Read the model definition and answer for the solid it produces. Units are mm, in the model's axes. A direction names the side the tool comes from. Give positions to 0.01 mm unless a question says otherwise; leave off trailing zeros. Order: outer loops, then holes, each group sorted by start corner. A loop starts at its lowest first (then second) coordinate and runs counter-clockwise, first axis right, second up. Notation, with made-up numbers: (88, -26) - (135, -26) arc R23 cw to (135, 5) - close; hole circle Ø2 at (11, 52.25). An arc over 180 degrees is marked (long way). Return JSON: item names as keys, results as strings.
```python
from build123d import *

# Parameters (mm, degrees)
F0_R     = 7.7179968939
F1_DEPTH = 38.1
F2_W     = 6.3499980524
F2_H     = 3.8099980524
F2_H_2   = 5.3974985393
F3_DEPTH = 12.7
F4_W     = 79.248
F4_H     = 25.4
F5_DEPTH = 44.45


with BuildPart() as f1:
    # F0 (on Front) → F1 (new body)
    with BuildSketch(Plane.XZ):
        Polygon((-13.60275174, 47.8438777382), (-35.95475174, 47.8438777382), (-35.95475174, 35.1438777382), (-55.00475174, 35.1438777382), (-55.00475174, -2.255679107), (36.94324826, -2.255679107), (18.8287593137, 29.1195361012), align=None)
        with Locations((-16.90475174, 23.144320893)):
            Circle(F0_R, mode=Mode.SUBTRACT)
    extrude(amount=F1_DEPTH)

    # F2 (on face) → F3 (join)
    with BuildSketch(Plane.XY.offset(35.1438777382)):
        with Locations((-45.4797527138, -29.8450009738)):
            Rectangle(F2_W, F2_H)
        with Locations((-45.4797527138, -9.0487492696)):
            Rectangle(F2_W, F2_H_2)
    extrude(amount=F3_DEPTH)

    # F4 (on face) → F5 (cut)
    with BuildSketch(Plane.XY.offset(47.8438777382)):
        with Locations((-9.03075174, -19.05)):
            Rectangle(F4_W, F4_H)
        Polygon((-42.3047536876, -27.9400019476), (-42.3047536876, -31.75), (30.59324826, -31.75), (30.59324826, -6.35), (-48.65475174, -6.35), (-48.65475174, -27.9400019476), align=None)
    extrude(amount=-F5_DEPTH, mode=Mode.SUBTRACT)


solid = f1.part
```
Q1. Determine the mould class of faces 1 (the flat face through (-25, -35, 47.844)), 2 (the cylindrical face through (-18.58, -34.88, 15.61)), 3 (the flat face through (-35.955, -3, 42)) for opening direction X: released by +X, released by -X, zero draft, split by the parting line, or undercut.
Values:
{"face 1": "zero draft", "face 2": "undercut", "face 3": "released by -X"}
Q2. For faces 4 (the flat face through (-10, -19, 3.394)), 5 (the flat face through (-50, -19, 35.144)), 6 (the flat face through (-10, -38.1, 18)), determine the directions among +Z, -Z, +X, -X, +Y, -Y from which every point of the face is accessible in a straight line to the end or side of a thin tool.
Values:
{"face 4": "+Z", "face 5": "+Z, -X, +Y, -Y", "face 6": "+Z, -Z, +X, -X, -Y"}
Q3. A cutting plane is placed at A-A (z = 20). Write down the section's boundary in (x, y), and give its area (3 significant figures).
Values:
{"outline": "(-55, -38.1) - (-23.95, -38.1) - (-23.95, -31.75) - (-48.65, -31.75) - (-48.65, -6.35) - (-23.95, -6.35) - (-23.95, 0) - (-55, 0) - close; (-9.86, -38.1) - (24.09, -38.1) - (24.09, -31.75) - (-9.86, -31.75) - close; (-9.86, -6.35) - (24.09, -6.35) - (24.09, 0) - (-9.86, 0) - close", "area": "987 mm²"}
Q4. Given pin 1 (5 mm diameter, centred on y = -3.5, z = 44.5, fed in from -X); pin 2 (12.5 mm diameter, centred on x = -16.9, z = 23.14, fed in from +Y); pin 3 (9.5 mm diameter, centred on x = -47, y = -13.5, fed in from +Z); pin 4 (3 mm diameter, centred on x = 17, y = -28.5, fed in from +Z), each flat-ended and moving along its own axis, determine where each tip first touches the part or whether it passes through.
Values:
{"pin 1": "stops at x = -35.95", "pin 2": "passes through", "pin 3": "stops at z = 35.14", "pin 4": "stops at z = 3.39"}
Q5. Consider L1, parallel to Y at x = 0, z = 6; L2, parallel to Z at x = 11, y = -28. Determine where each line is inside the solid, lowest interval first.
Values:
{"L1": "y = -38.1 to -31.75, -6.35 to 0", "L2": "z = -2.26 to 3.39"}
Q6. A cutting plane is placed at D-D (z = 37). Write down the section's boundary in (x, y).
Values:
{"outline": "(-35.95, -38.1) - (5.18, -38.1) - (5.18, -31.75) - (-35.95, -31.75) - close; (-35.95, -6.35) - (5.18, -6.35) - (5.18, 0) - (-35.95, 0) - close"}
Q7. A cutting plane is placed at C-C (x = -27.5). Write down the section's boundary in (y, z).
Values:
{"outline": "(-38.1, -2.26) - (0, -2.26) - (0, 47.84) - (-6.35, 47.84) - (-6.35, 3.39) - (-31.75, 3.39) - (-31.75, 47.84) - (-38.1, 47.84) - close"}
Q8. A cutting plane is placed at B-B (y = -2.5). Write down the section's boundary in (x, z), and give its area (3 significant figures).
Values:
{"outline": "(-55, -2.26) - (36.94, -2.26) - (18.83, 29.12) - (-13.6, 47.84) - (-35.95, 47.84) - (-35.95, 35.14) - (-55, 35.14) - close; hole circle Ø15.44 at (-16.9, 23.14)", "area": "3,250 mm²"}
